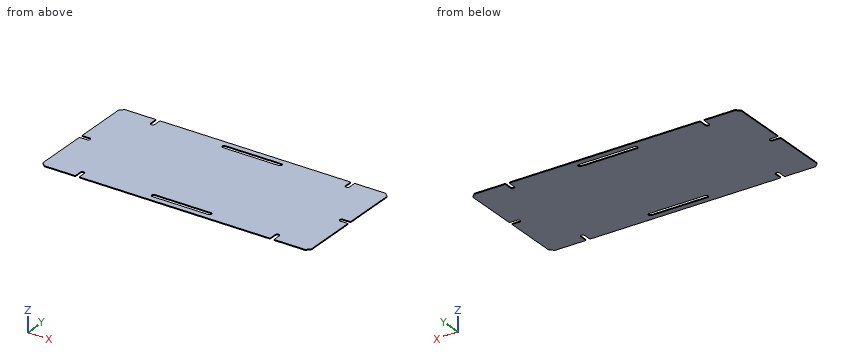
```python
from build123d import *

# Parameters (mm, degrees)
SKETCH1_W                   = 455.168
SKETCH1_H                   = 201.168
BOSS_EXTRUDE1_DEPTH         = 1.5875
F_1_4_CLEARANCE_HOLE1_D     = 6.7564
F_1_4_CLEARANCE_SLOT1_DEPTH = 1.5875
CHAMFER1_SIZE               = 6.35
CUT_EXTRUDE1_REACH          = 250.826
SKETCH6_W                   = 6.7564
SKETCH6_H                   = 14.478
CUT_EXTRUDE2_REACH          = 250.826
SKETCH7_W                   = 14.478
SKETCH7_H                   = 6.7564


# Read off the part's stored shape, not the designer's step: 1/4 Clearance Slot1
with BuildPart() as part:
    # Sketch1 → Boss-Extrude1 (new body)
    with BuildSketch(Plane.XY):
        Rectangle(SKETCH1_W, SKETCH1_H)
    extrude(amount=BOSS_EXTRUDE1_DEPTH)

    # 1/4 Clearance Hole1 (through all)
    with Locations(Plane.XY.offset(1.5875)):
        with Locations((-165.1, 87.884), (165.1, 87.884), (214.884, 0), (-214.884, 0), (-165.1, -87.884), (165.1, -87.884)):
            Hole(F_1_4_CLEARANCE_HOLE1_D / 2)

    # 1/4 Clearance Slot1 outline → 1/4 Clearance Slot1 (cut)
    with BuildSketch(Plane.XY):
        with BuildLine():
            Line((-44.1706, 84.5058), (50.673, 84.5058))
            ThreePointArc((50.673, 84.5058), (54.0512, 87.884), (50.673, 91.2622))
            Line((50.673, 91.2622), (-44.1706, 91.2622))
            ThreePointArc((-44.1706, 91.2622), (-47.5488, 87.884), (-44.1706, 84.5058))
        make_face()
        with BuildLine():
            Line((-44.1706, -91.2622), (50.673, -91.2622))
            ThreePointArc((50.673, -91.2622), (54.0512, -87.884), (50.673, -84.5058))
            Line((50.673, -84.5058), (-44.1706, -84.5058))
            ThreePointArc((-44.1706, -84.5058), (-47.5488, -87.884), (-44.1706, -91.2622))
        make_face()
    extrude(amount=F_1_4_CLEARANCE_SLOT1_DEPTH, mode=Mode.SUBTRACT)

    # Chamfer1
    chamfer1_edges = [part.edges().sort_by_distance(p)[0] for p in [
        (227.584, -100.584, 0.79375),
        (-227.584, -100.584, 0.79375),
        (-227.584, 100.584, 0.79375),
        (227.584, 100.584, 0.79375),
    ]]
    chamfer(chamfer1_edges, length=CHAMFER1_SIZE)

    # Sketch6 → Cut-Extrude1 (cut, up to next)
    with BuildSketch(Plane.XY.offset(1.5875), mode=Mode.PRIVATE) as cut_extrude1_sk1:
        with Locations((-165.1, 95.123)):
            Rectangle(SKETCH6_W, SKETCH6_H)
    cut_extrude1_tool1 = extrude(cut_extrude1_sk1.sketch, amount=-CUT_EXTRUDE1_REACH, mode=Mode.PRIVATE) & part.part
    # Sketch6 → Cut-Extrude1 (cut, up to next)
    with BuildSketch(Plane.XY.offset(1.5875), mode=Mode.PRIVATE) as cut_extrude1_sk2:
        with Locations((165.1, 95.123)):
            Rectangle(SKETCH6_W, SKETCH6_H)
    cut_extrude1_tool2 = extrude(cut_extrude1_sk2.sketch, amount=-CUT_EXTRUDE1_REACH, mode=Mode.PRIVATE) & part.part
    cut_extrude1_1 = cut_extrude1_tool1.solids().sort_by_distance((-165.1, 95.123, 1.5875))[0]
    add(cut_extrude1_1, mode=Mode.SUBTRACT)
    cut_extrude1_2 = cut_extrude1_tool2.solids().sort_by_distance((165.1, 95.123, 1.5875))[0]
    add(cut_extrude1_2, mode=Mode.SUBTRACT)
    cut_extrude1 = cut_extrude1_1 + cut_extrude1_2  # Cut-Extrude1 as one shape, for the pattern or mirror that repeats it

    # Mirror1: Cut-Extrude1 across plane
    add(cut_extrude1.mirror(Plane.ZX), mode=Mode.SUBTRACT)

    # Sketch7 → Cut-Extrude2 (cut, up to next)
    with BuildSketch(Plane.XY.offset(1.5875), mode=Mode.PRIVATE) as cut_extrude2_sk1:
        with Locations((-222.123, 0)):
            Rectangle(SKETCH7_W, SKETCH7_H)
    cut_extrude2_tool1 = extrude(cut_extrude2_sk1.sketch, amount=-CUT_EXTRUDE2_REACH, mode=Mode.PRIVATE) & part.part
    cut_extrude2 = cut_extrude2_tool1.solids().sort_by_distance((-222.123, 0, 1.5875))[0]
    add(cut_extrude2, mode=Mode.SUBTRACT)

    # Mirror2: Cut-Extrude2 across plane
    add(cut_extrude2.mirror(Plane(origin=(0, 0, 0), x_dir=(0, 0, 1), z_dir=(1, 0, 0))), mode=Mode.SUBTRACT)


solid = part.part
```
Could you check a few things on this model? Use its own coordinates, in mm. Coordinates: 2 decimals unless noted, no trailing zeros. Write each loop counter-clockwise with the first axis right and the second up, starting at its lowest first coordinate (ties: lowest second). Pieces come first, ordered by that corner, then holes. Notation, with made-up numbers: (72, -20.75) -> (78, -20.75) arc R19 ccw to (78, -16.75) -> close; hole circle Ø9 at (55.25, 39). An arc over 180 degrees is marked (long way). Write item = value, one per line. Start each with the question number.
(1) Will this pin go through, and if not, where does the flat tip stop? pin 1 (0.8 mm diameter, centred on y = -95, z = 1, fed in from +X).
(2) I want a section at A-A (x = -38). Please give me the cut outline in (y, z).
(3) I want a section at B-B (z = 0.8). Give the number of separate pieces and of enclosed holes in the cut face, plus the area to 3 significant figures.
(4) I need wall thicknesses on line 1 (Y direction, x = 20, z = 1.5); line 2 (X direction, y = -88, z = 1.4); line 3 (X direction, y = 90, z = 1.45). Which ranges of each line are inside material? Lowest first, please. Write a range as [from, to].
Result set:
q1.pin_1 = 227.22
q2.outline = (-100.58, 0) -> (-91.26, 0) -> (-91.26, 1.59) -> (-100.58, 1.59) -> close; (-84.51, 0) -> (84.51, 0) -> (84.51, 1.59) -> (-84.51, 1.59) -> close; (91.26, 0) -> (100.58, 0) -> (100.58, 1.59) -> (91.26, 1.59) -> close
q3.separate_pieces = 1
q3.enclosed_holes = 2
q3.area = 89,500 mm2
q4.line_1 = [-100.58, -91.26], [-84.51, 84.51], [91.26, 100.58]
q4.line_2 = [-227.58, -168.48], [-161.72, -47.55], [54.05, 161.72], [168.48, 227.58]
q4.line_3 = [-227.58, -168.48], [-161.72, -46.8], [53.31, 161.72], [168.48, 227.58]
